Here's how the part is built. I have some questions about the finished solid (model axes, mm). A direction names the side the tool comes from. Round coordinates to 2 decimals unless told otherwise and drop trailing zeros. Write each loop counter-clockwise with the first axis right and the second up, starting at its lowest first coordinate (ties: lowest second). Pieces come first, ordered by that corner, then holes. Notation, with made-up numbers: M -20.5,-32 L -11.5,-32 A32 cw -11.5,3 Z; hole C -5,4 d6. An arc over 180 degrees is marked long. Write item = value, one per line. Start each with the question number.
(1) If we mould it in two halves opening along Y, with no side actions, what happens to faces 1 (the cylindrical face through (-57.71, -37.23, 1.48)), 2 (the cylindrical face through (-9.693, 46.514, 4.972)), 3 (the flat face through (-53, -12, 7)), 4 (the flat face through (-30, 65.868, 1))? For each: released by +Y, released by -Y, zero draft, split by the parting line, or undercut.
(2) I need wall thicknesses on line 1 along Y through (x, z) = (-11.5, 0.5); line 2 along Y through (x, z) = (-54.5, 6); line 3 along Z through (x, y) = (-32, 51). Which ranges of each line are inside material? Lowest first, please.
(3) I want a section at C-C (y = 1.5). List the corners of the cut face in (x, z) for me, and give its area (3 significant figures).
(4) Will these pins go through, and if not, where does the flat tip stop? pin 1 Ø3.5 at (x, y) = (-10.57, 35.87) entering from +Z; pin 2 Ø4 at (x, y) = (-55.07, 46.37) entering from +Z; pin 3 Ø1.7 at (x, y) = (-55.07, 46.37) entering from +Z.
(5) I want a section at B-B (x = -45). List the corners of the cut face in (y, z) for me, and give its area (3 significant figures).
(6) I want a section at A-A (z = 5). List the corners of the cut face in (x, y) for me.
(7) On a 3-axis mill with a long thin cutter (end or side, diameter ignored), from which of +Z, -Z, +X, -X, +Y, -Y can I reach the whole of each face in a straight line? I mean faces 5 (the cylindrical face through (-9.693, -11.486, 4.972)), 6 (the flat face through (-58.567, 16, 1)). Say none if no direction works.
```python
from build123d import *

# Parameters (mm, degrees)
BOSS_EXTRUDE1_DEPTH = 3
SKETCH3_R           = 1.6
SKETCH3_R_2         = 1.45
CUT_EXTRUDE1_DEPTH  = 4
SKETCH4_R           = 1.45
BOSS_EXTRUDE2_DEPTH = 4


with BuildPart() as part:
    # Sketch2 → Boss-Extrude1 (new body)
    with BuildSketch(Plane.XY):
        with BuildLine():
            Line((-55.566838563, -38.131712133), (-5.566838563, -38.131712133))
            ThreePointArc((-5.566838563, -38.131712133), (-3.44551822, -37.253032477), (-2.566838563, -35.131712133))
            Line((-2.566838563, -35.131712133), (-2.566838563, 65.868287867))
            Line((-2.566838563, 65.868287867), (-58.566838563, 65.868287867))
            Line((-58.566838563, 65.868287867), (-58.566838563, -35.131712133))
            ThreePointArc((-58.566838563, -35.131712133), (-57.688158907, -37.253032477), (-55.566838563, -38.131712133))
        make_face()
    extrude(amount=BOSS_EXTRUDE1_DEPTH)

    # Sketch3 → Cut-Extrude1 (cut, through all)
    with BuildSketch(Plane.XY.offset(3)):
        with Locations((-50.566838563, 35.868287867)):
            Circle(SKETCH3_R)
        with Locations((-50.566838563, 5.868287867)):
            Circle(SKETCH3_R)
        with Locations((-10.566838563, 5.868287867)):
            Circle(SKETCH3_R)
        with Locations((-10.566838563, 35.868287867)):
            Circle(SKETCH3_R)
        with Locations((-40.566838563, 24.968287867)):
            Circle(SKETCH3_R_2)
        with Locations((-15.166838563, -30.231712133)):
            Circle(SKETCH3_R_2)
        with Locations((-6.066838563, 46.368287867)):
            Circle(SKETCH3_R_2)
        with Locations((-6.066838563, -11.631712133)):
            Circle(SKETCH3_R_2)
        with Locations((-55.066838563, -11.631712133)):
            Circle(SKETCH3_R_2)
        with Locations((-55.066838563, 46.368287867)):
            Circle(SKETCH3_R_2)
    extrude(amount=-CUT_EXTRUDE1_DEPTH, mode=Mode.SUBTRACT)

    # Sketch4 → Boss-Extrude2 (add)
    with BuildSketch(Plane.XY.offset(3)):
        with BuildLine():
            Line((-58.566838563, -10.671563034), (-58.566838563, -12.591861232))
            ThreePointArc((-58.566838563, -12.591861232), (-54.582429852, -15.228548867), (-51.437529223, -11.631712133))
            ThreePointArc((-51.437529223, -11.631712133), (-54.582429852, -8.034875399), (-58.566838563, -10.671563034))
        make_face()
        with Locations((-55.066838563, -11.631712133)):
            Circle(SKETCH4_R, mode=Mode.SUBTRACT)
        with BuildLine():
            Line((-58.566838563, 47.328436966), (-58.566838563, 45.408138768))
            ThreePointArc((-58.566838563, 45.408138768), (-54.582429852, 42.771451133), (-51.437529223, 46.368287867))
            ThreePointArc((-51.437529223, 46.368287867), (-54.582429852, 49.965124601), (-58.566838563, 47.328436966))
        make_face()
        with Locations((-55.066838563, 46.368287867)):
            Circle(SKETCH4_R, mode=Mode.SUBTRACT)
        with BuildLine():
            ThreePointArc((-2.566838563, -10.671563034), (-9.696147904, -11.631712133), (-2.566838563, -12.591861232))
            Line((-2.566838563, -12.591861232), (-2.566838563, -10.671563034))
        make_face()
        with Locations((-6.066838563, -11.631712133)):
            Circle(SKETCH4_R, mode=Mode.SUBTRACT)
        with BuildLine():
            ThreePointArc((-2.566838563, 47.328436966), (-9.696147904, 46.368287867), (-2.566838563, 45.408138768))
            Line((-2.566838563, 45.408138768), (-2.566838563, 47.328436966))
        make_face()
        with Locations((-6.066838563, 46.368287867)):
            Circle(SKETCH4_R, mode=Mode.SUBTRACT)
    extrude(amount=BOSS_EXTRUDE2_DEPTH)


solid = part.part
```
Returned:
q1.face_1 = released by -Y
q1.face_2 = undercut
q1.face_3 = zero draft
q1.face_4 = released by +Y
q2.line_1 = -38.13 to 4.57, 7.17 to 34.57, 37.17 to 65.87
q2.line_2 = -15.22 to -12.97, -10.3 to -8.05, 42.78 to 45.03, 47.7 to 49.95
q2.line_3 = 0 to 3
q3.outline = M -58.57,0 L -2.57,0 L -2.57,3 L -58.57,3 Z
q3.area = 168 mm²
q4.pin_1 = 3
q4.pin_2 = 7
q4.pin_3 = through
q5.outline = M -38.13,0 L 65.87,0 L 65.87,3 L -38.13,3 Z
q5.area = 312 mm²
q6.outline = M -58.57,-12.59 A3.63 ccw long -58.57,-10.67 Z; M -58.57,45.41 A3.63 ccw long -58.57,47.33 Z; M -2.57,-12.59 L -2.57,-10.67 A3.63 ccw long Z; M -2.57,45.41 L -2.57,47.33 A3.63 ccw long Z; hole C -55.07,-11.63 d2.9; hole C -55.07,46.37 d2.9; hole C -6.07,-11.63 d2.9; hole C -6.07,46.37 d2.9
q7.face_5 = +Z
q7.face_6 = +Z, -Z, -X, +Y, -Y
